```python
from build123d import *

# Parameters (mm, degrees)
F0_W          = 530
F0_H          = 530
F0_R          = 250
F1_DEPTH      = 65
F1_DEPTH_BACK = 65
F2_R          = 10
F3_DEPTH      = 12
F3_DEPTH_BACK = 542
F4_R          = 150
F0_R_2        = 110
F5_DEPTH      = 211
F5_DEPTH_BACK = 211
F6_DEPTH      = 171
F6_DEPTH_BACK = 171
F7_SIZE2      = 69.282022
F7_SIZE       = 39.99999
F8_SIZE2      = 69.282022
F8_SIZE       = 39.99999


# Not quite as in the source:
# - a fillet or chamfer is up to 0.001 mm smaller than in the source, because OpenCascade refuses the exact size


with BuildPart() as f1:
    # F0 (on Front) → F1 (new body, two sides)
    with BuildSketch(Plane.XZ) as f1_sk:
        Rectangle(F0_W, F0_H)
        Circle(F0_R, mode=Mode.SUBTRACT)
    extrude(amount=F1_DEPTH)
    extrude(f1_sk.sketch, amount=-F1_DEPTH_BACK)

    # F2 (on face) → F3 (join, two sides)
    with BuildSketch(Plane.YZ.offset(265)) as f3_sk:
        with Locations((-45, 90)):
            Circle(F2_R)
        with Locations((45, 90)):
            Circle(F2_R)
        with Locations((45, -90)):
            Circle(F2_R)
        with Locations((-45, -90)):
            Circle(F2_R)
    extrude(amount=F3_DEPTH)
    extrude(f3_sk.sketch, amount=-F3_DEPTH_BACK)

    # F4
    f4_edges = [f1.edges().sort_by_distance(p)[0] for p in [
        (265, 0, 265),
        (-265, 0, 265),
        (265, 0, -265),
        (-265, 0, -265),
    ]]
    fillet(f4_edges, radius=F4_R)

    # F0 (on Front) → F5 (join, two sides)
    with BuildSketch(Plane.XZ) as f5_sk:
        Circle(F0_R)
        Circle(F0_R_2, mode=Mode.SUBTRACT)
    extrude(amount=F5_DEPTH)
    extrude(f5_sk.sketch, amount=-F5_DEPTH_BACK)

    # F0 (on Front) → F6 (join, two sides)
    with BuildSketch(Plane.XZ) as f6_sk:
        Circle(F0_R_2)
    extrude(amount=F6_DEPTH)
    extrude(f6_sk.sketch, amount=-F6_DEPTH_BACK)

    # F7 (size 40 and 69.2820323028 in the source; OpenCascade refuses exactly that, so slightly less here)
    f7_edges = [f1.edges().sort_by_distance(p)[0] for p in [
        (-110, -211, 0),
    ]]
    f7_side = f1.faces().sort_by_distance((-110, -191, 0))[0]
    chamfer(f7_edges, length=F7_SIZE, length2=F7_SIZE2, reference=f7_side)

    # F8 (size 40 and 69.2820323028 in the source; OpenCascade refuses exactly that, so slightly less here)
    f8_edges = [f1.edges().sort_by_distance(p)[0] for p in [
        (-110, 211, 0),
    ]]
    f8_side = f1.faces().sort_by_distance((-110, 191, 0))[0]
    chamfer(f8_edges, length=F8_SIZE, length2=F8_SIZE2, reference=f8_side)


solid = f1.part
```
Here's how the part is built. I have some questions about the finished solid (model axes, mm). A direction names the side the tool comes from. Round coordinates to 2 decimals unless told otherwise and drop trailing zeros. Order: outer loops, then holes, each group sorted by start corner. A loop starts at its lowest first (then second) coordinate and runs counter-clockwise, first axis right, second up. Notation, with made-up numbers: M 85.25,56 L 91.25,56 A23 cw 91.25,76 Z; hole C -1,-12.5 d9. An arc over 180 degrees is marked long. Answer as CSV lines item,"result".
Item 1: Please list where these lines run through material, in increasing order: L1, parallel to Z at x = 0, y = 171.05; L2, parallel to X at y = 32.5, z = 45; L3, parallel to Y at x = -211, z = -153.5. Write a range as [from, to].
From the geometry:
L1,"[-250, -110.09], [110.09, 250]"
L2,"[-265, 265]"
L3,"[-65, 65]"
Item 2: Imagine slicing it at A-A on y = -45. List the corners of the cut face in (x, z) for me, and give its area (3 significant figures).
From the geometry:
outline,"M -277,-100 L -265,-100 L -265,-115 A150 ccw -115,-265 L 115,-265 A150 ccw 265,-115 L 265,-100 L 277,-100 L 277,-80 L 265,-80 L 265,80 L 277,80 L 277,100 L 265,100 L 265,115 A150 ccw 115,265 L -115,265 A150 ccw -265,115 L -265,100 L -277,100 L -277,80 L -265,80 L -265,-80 L -277,-80 Z"
area,"263,000 mm2"
Item 3: Imagine slicing it at C-C on z = -205.5. List the corners of the cut face in (x, y) for me.
From the geometry:
outline,"M -234.62,-65 L -142.37,-65 L -142.37,-211 L 142.37,-211 L 142.37,-65 L 234.62,-65 L 234.62,65 L 142.37,65 L 142.37,211 L -142.37,211 L -142.37,65 L -234.62,65 Z"
Item 4: For pin 1 (1 mm diameter, centred on x = -83.5, y = 144, fed in from +Z); pin 2 (4 mm diameter, centred on x = -192.5, z = 209.5, fed in from +Y); pin 3 (8 mm diameter, centred on x = -53, y = 74, fed in from -Z), each with a flat end and sliding along its axis, tell me the tip position at first contact or that it passes through.
From the geometry:
pin 1,"z = 235.82"
pin 2,"y = 65"
pin 3,"z = -245.15"
Item 5: Which directions (+Z, -Z, +X, -X, +Y, -Y) give clear straight access to the entire face, cutting with the end or side of a thin tool? Please do faces 1 (the cylindrical face through (-270.916, -46.302, 99.915)), 2 (the flat face through (-2, -171, 2)), 3 (the flat face through (-2, -1, -265)), 4 (the cylindrical face through (-249.76, 136.98, 10.99)), 5 (the cylindrical face through (270.916, -46.302, 99.915)).
From the geometry:
face 1,"-X"
face 2,"-Y"
face 3,"-Z, +X, -X, +Y, -Y"
face 4,"+Y"
face 5,"+X"
Item 6: We'd pull the mould along Z, two halves only. Please class faces 6 (the flat face through (-2, 171, 2)), 7 (the flat face through (277, -45, -90)), 8 (the cylindrical face through (-249.76, -136.98, 10.99)): +Z half, -Z half, draft (parallel to the pull), parting line (faces both ways), or undercut.
From the geometry:
face 6,"undercut"
face 7,"draft"
face 8,"parting line"
Item 7: Imagine slicing it at D-D on x = -242. List the corners of the cut face in (y, z) for me, and give its area (3 significant figures).
From the geometry:
outline,"M -211,-62.74 L -65,-62.74 L -65,-194.82 L 65,-194.82 L 65,-62.74 L 211,-62.74 L 211,62.74 L 65,62.74 L 65,194.82 L -65,194.82 L -65,62.74 L -211,62.74 Z"
area,"87,300 mm2"
